from build123d import *

# Parameters (mm, degrees)
BOSS_EXTRUDE1_DEPTH = 43
CUT_EXTRUDE1_REACH  = 69.604
SKETCH2_R           = 1.25
FILLET1_R           = 2.5
FILLET2_R           = 2.5
FILLET3_R           = 1
FILLET4_R           = 1


with BuildPart() as part:
    # Sketch1 → Boss-Extrude1 (new body)
    with BuildSketch(Plane.XY):
        Polygon((0, 0), (1.6, 31.458886043), (31.6, 31.458886043), (33.6, -28.041113957), (36.6, -28.041113957), (36.6, 33.958886043), (-3, 33.958886043), (-3, 0), align=None)
    extrude(amount=-BOSS_EXTRUDE1_DEPTH)

    # Cut-Extrude1: up to this plane
    cut_extrude1_end = Plane(origin=(31.6, 31.458886043, -43), z_dir=(-0.9994355464166094, -0.03359447214845748, 0))
    # Sketch2 → Cut-Extrude1 (cut, up to the surface)
    with BuildSketch(Plane(origin=(36.6, 0, 0), x_dir=(0, 0, -1), z_dir=(1, 0, 0)), mode=Mode.PRIVATE) as cut_extrude1_sk1:
        with Locations(Location((39.25, 17.819052722, 0), (0, 0, 90))):
            Circle(SKETCH2_R)
    cut_extrude1_tool1 = split(extrude(cut_extrude1_sk1.sketch, amount=-CUT_EXTRUDE1_REACH, mode=Mode.PRIVATE), bisect_by=cut_extrude1_end, keep=Keep.BOTH, mode=Mode.PRIVATE)
    add(cut_extrude1_tool1.solids().sort_by_distance((36.6, 17.819053, -39.25))[0], mode=Mode.SUBTRACT)
    # Sketch2 → Cut-Extrude1 (cut, up to the surface)
    with BuildSketch(Plane(origin=(36.6, 0, 0), x_dir=(0, 0, -1), z_dir=(1, 0, 0)), mode=Mode.PRIVATE) as cut_extrude1_sk2:
        with Locations(Location((39.25, -4.180947278, 0), (0, 0, 90))):
            Circle(SKETCH2_R)
    cut_extrude1_tool2 = split(extrude(cut_extrude1_sk2.sketch, amount=-CUT_EXTRUDE1_REACH, mode=Mode.PRIVATE), bisect_by=cut_extrude1_end, keep=Keep.BOTH, mode=Mode.PRIVATE)
    add(cut_extrude1_tool2.solids().sort_by_distance((36.6, -4.180947, -39.25))[0], mode=Mode.SUBTRACT)
    # Sketch2 → Cut-Extrude1 (cut, up to the surface)
    with BuildSketch(Plane(origin=(36.6, 0, 0), x_dir=(0, 0, -1), z_dir=(1, 0, 0)), mode=Mode.PRIVATE) as cut_extrude1_sk3:
        with Locations(Location((3.75, -4.180947278, 0), (0, 0, 270))):
            Circle(SKETCH2_R)
    cut_extrude1_tool3 = split(extrude(cut_extrude1_sk3.sketch, amount=-CUT_EXTRUDE1_REACH, mode=Mode.PRIVATE), bisect_by=cut_extrude1_end, keep=Keep.BOTH, mode=Mode.PRIVATE)
    add(cut_extrude1_tool3.solids().sort_by_distance((36.6, -4.180947, -3.75))[0], mode=Mode.SUBTRACT)
    # Sketch2 → Cut-Extrude1 (cut, up to the surface)
    with BuildSketch(Plane(origin=(36.6, 0, 0), x_dir=(0, 0, -1), z_dir=(1, 0, 0)), mode=Mode.PRIVATE) as cut_extrude1_sk4:
        with Locations(Location((3.75, 17.819052722, 0), (0, 0, 270))):
            Circle(SKETCH2_R)
    cut_extrude1_tool4 = split(extrude(cut_extrude1_sk4.sketch, amount=-CUT_EXTRUDE1_REACH, mode=Mode.PRIVATE), bisect_by=cut_extrude1_end, keep=Keep.BOTH, mode=Mode.PRIVATE)
    add(cut_extrude1_tool4.solids().sort_by_distance((36.6, 17.819053, -3.75))[0], mode=Mode.SUBTRACT)

    # Fillet1
    fillet1_edges = [part.edges().sort_by_distance(p)[0] for p in [
        (31.6, 31.458886043, -21.5),
        (1.6, 31.458886043, -21.5),
    ]]
    fillet(fillet1_edges, radius=FILLET1_R)

    # Fillet2
    fillet2_edges = [part.edges().sort_by_distance(p)[0] for p in [
        (-3, 33.958886043, -21.5),
        (36.6, 33.958886043, -21.5),
    ]]
    fillet(fillet2_edges, radius=FILLET2_R)

    # Fillet3
    fillet3_edges = [part.edges().sort_by_distance(p)[0] for p in [
        (-1.5, 0, 0),
        (-3, 0, -21.5),
        (0, 0, -21.5),
        (-1.5, 0, -43),
    ]]
    fillet(fillet3_edges, radius=FILLET3_R)

    # Fillet4
    fillet4_edges = [part.edges().sort_by_distance(p)[0] for p in [
        (36.6, -28.041113957, -21.5),
        (33.6, -28.041113957, -21.5),
        (35.1, -28.041113957, -43),
        (35.1, -28.041113957, 0),
    ]]
    fillet(fillet4_edges, radius=FILLET4_R)


solid = part.part
Design review of the part built by this model. Coordinates are the model's own, in mm. A direction names the side the tool comes from. Coordinates: 2 decimals unless noted, no trailing zeros. Write each loop counter-clockwise with the first axis right and the second up, starting at its lowest first coordinate (ties: lowest second). Pieces come first, ordered by that corner, then holes. Notation, with made-up numbers: (-16, -11.5) - (30, -11.5) arc R15 cw to (30, 7.5) - close; hole circle Ø1 at (62, -14). An arc over 180 degrees is marked (long way). One line per item, written item: value.
1) Insertion check: pin 1 (8 mm diameter, centred on x = 14, z = -25.5, fed in from -Y); pin 2 (1.2 mm diameter, centred on x = -1.5, z = -18, fed in from -Y). Each pin has a flat end and moves straight along its axis. Give the tip position at first contact, or say it passes through.
Answer sheet:
pin 1: stops at y = 31.46
pin 2: stops at y = 0
2) Add section A-A (y = 15.5). State the section outline as (x, z) points.
Answer sheet:
outline: (-3, -43) - (0.79, -43) - (0.79, 0) - (-3, 0) - close; (32.14, -43) - (36.6, -43) - (36.6, 0) - (32.14, 0) - close
3) Mouldability with a two-part tool opening along Y and no side actions: class faces 4 (the face through (17, 33.959, -21)), 5 (the face through (34.7, -4.76, -2.64)), 6 (the face through (34.34, 16.664, -3.271)), 7 (the face through (33, 15, -43)) as +Y half, -Y half, draft (parallel to the pull), parting line (faces both ways), or undercut.
Answer sheet:
face 4: +Y half
face 5: undercut
face 6: undercut
face 7: draft
4) To check wall thickness, follow probe 1 along Y at (x, z) = (10, -14.5); probe 2 along X at (y, z) = (28, -33); probe 3 along X at (y, z) = (23.5, -23). State the ranges of each line that lie inside material, in increasing order.
Answer sheet:
probe 1: y = 31.46 to 33.96
probe 2: x = -3 to 1.42, 31.72 to 36.6
probe 3: x = -3 to 1.2, 31.87 to 36.6
5) Add section C-C (z = -3.75). State the section outline as (x, y) points.
Answer sheet:
outline: (-3, 1) arc R1 ccw to (-2, 0) - (-0.95, 0) arc R1 ccw to (0.05, 0.95) - (1.48, 29.09) arc R2.5 cw to (3.98, 31.46) - (29.18, 31.46) arc R2.5 cw to (31.68, 29.04) - (32.02, 19.07) - (36.6, 19.07) - (36.6, 31.46) arc R2.5 ccw to (34.1, 33.96) - (-0.5, 33.96) arc R2.5 ccw to (-3, 31.46) - close; (32.1, 16.57) - (32.76, -2.93) - (36.6, -2.93) - (36.6, 16.57) - close; (32.84, -5.43) - (33.57, -27.07) arc R1 ccw to (34.57, -28.04) - (35.6, -28.04) arc R1 ccw to (36.6, -27.04) - (36.6, -5.43) - close
6) Add section D-D (y = 28). State the section outline as (x, z) points, plus the area to 3 significant figures.
Answer sheet:
outline: (-3, -43) - (1.42, -43) - (1.42, 0) - (-3, 0) - close; (31.72, -43) - (36.6, -43) - (36.6, 0) - (31.72, 0) - close
area: 400 mm2
7) For faces 1 (the face through (2.23, 30.75, -21.8)), 2 (the face through (34.7, -4.34, -38.01)), 3 (the face through (34.34, 16.57, -39.2)), list the 3-axis set-ups (+Z, -Z, +X, -X, +Y, -Y) from which the entire face can be reached by the end or side of a thin tool; tool diameter is ignored.
Answer sheet:
face 1: +Z, -Z, -Y
face 2: +X, -X
face 3: +X
8) Add section B-B (z = -37). State the section outline as (x, y) points, plus the area to 3 significant figures.
Answer sheet:
outline: (-3, 1) arc R1 ccw to (-2, 0) - (-0.95, 0) arc R1 ccw to (0.05, 0.95) - (1.48, 29.09) arc R2.5 cw to (3.98, 31.46) - (29.18, 31.46) arc R2.5 cw to (31.68, 29.04) - (33.57, -27.07) arc R1 ccw to (34.57, -28.04) - (35.6, -28.04) arc R1 ccw to (36.6, -27.04) - (36.6, 31.46) arc R2.5 ccw to (34.1, 33.96) - (-0.5, 33.96) arc R2.5 ccw to (-3, 31.46) - close
area: 455 mm2
